Source: CAD feature listing. Evaluate the final solid. Frame: model axes, mm. A direction names the side the tool comes from. Give positions to 0.01 mm unless a question says otherwise; leave off trailing zeros. Order: outer loops, then holes, each group sorted by start corner. A loop starts at its lowest first (then second) coordinate and runs counter-clockwise, first axis right, second up. Notation, with made-up numbers: M -38,71 L 3,71 A19 cw 3,103 Z; hole C 79,81.25 d3. An arc over 180 degrees is marked long. One line per question, with ' | ' between items. Start each with the question number.
from build123d import *

# Parameters (mm, degrees)
RESSALTO_EXTRUS_O1_DEPTH = 5
ESBO_O2_R                = 1.5
CORTE_EXTRUS_O1_DEPTH    = 5
FILETE1_R                = 10
CORTE_EXTRUS_O2_DEPTH    = 5
FILETE2_R                = 5


with BuildPart() as part:
    # Esboço1 → Ressalto-extrusão1 (new body)
    with BuildSketch(Plane.XY):
        with BuildLine():
            Line((-14.089663978, 13.135393664), (-14.089663978, 28.135393664))
            Line((-14.089663978, 28.135393664), (-34.089663978, 28.135393664))
            Line((-34.089663978, 28.135393664), (-34.089663978, 128.135393664))
            Line((-34.089663978, 128.135393664), (25.910336022, 128.135393664))
            Line((25.910336022, 128.135393664), (25.910336022, 28.135393664))
            Line((25.910336022, 28.135393664), (5.910336022, 28.135393664))
            Line((5.910336022, 28.135393664), (5.910336022, 13.135393664))
            ThreePointArc((5.910336022, 13.135393664), (-4.089663978, 3.135393664), (-14.089663978, 13.135393664))
        make_face()
    extrude(amount=RESSALTO_EXTRUS_O1_DEPTH)

    # Esboço2 → Corte-extrusão1 (cut)
    with BuildSketch(Plane.XY.offset(5)):
        with Locations((-4.089663978, 13.135393664)):
            Circle(ESBO_O2_R)
    extrude(amount=-CORTE_EXTRUS_O1_DEPTH, mode=Mode.SUBTRACT)

    # Filete1
    filete1_edges = [part.edges().sort_by_distance(p)[0] for p in [
        (5.910336022, 28.135393664, 2.5),
        (-14.089663978, 28.135393664, 2.5),
    ]]
    fillet(filete1_edges, radius=FILETE1_R)
    filete1_2_edges = [part.edges().sort_by_distance(p)[0] for p in [
        (25.910336022, 28.135393664, 2.5),
        (-34.089663978, 28.135393664, 2.5),
    ]]
    fillet(filete1_2_edges, radius=FILETE1_R - 0.0001)  # a hair under: the kernel refuses the full size

    # Esboço3 → Corte-extrusão2 (cut)
    with BuildSketch(Plane.XY.offset(5)):
        with BuildLine():
            ThreePointArc((-34.089663978, 38.135393664), (-27.631189305, 83.135393664), (-34.089663978, 128.135393664))
            Line((-34.089663978, 128.135393664), (-34.089663978, 38.135393664))
        make_face()
        with BuildLine():
            ThreePointArc((25.910336022, 38.135393664), (19.45186135, 83.135393664), (25.910336022, 128.135393664))
            Line((25.910336022, 128.135393664), (25.910336022, 38.135393664))
        make_face()
    extrude(amount=-CORTE_EXTRUS_O2_DEPTH, mode=Mode.SUBTRACT)

    # Filete2
    filete2_edges = [part.edges().sort_by_distance(p)[0] for p in [
        (-34.089663978, 128.135393664, 2.5),
        (25.910336022, 128.135393664, 2.5),
    ]]
    fillet(filete2_edges, radius=FILETE2_R)


solid = part.part
Item 1: Pin query (flat end, axial travel): pin 1 Ø3.5 at (x, y) = (-4.09, 13.14) entering from -Z; pin 2 Ø3 at (y, z) = (55, 1.5) entering from -X. Return the tip coordinate at first contact, or that it passes through.
Item 2: Cut plane D-D on x = 9.5. Return the cut outline in (y, z).
Item 3: Mould query, pull axis Y, two halves, no side actions, for faces 4 (the flat face through (-4, 80, 0)), 5 (the cylindrical face through (-27.677, 79.324, 2.535)), 6 (the cylindrical face through (-31.083, 30.987, 2.535)), 7 (the cylindrical face through (19.497, 79.324, 2.535)). Classes: pulls with the +Y half, pulls with the -Y half, needs draft (parallel to the pull), parting line crosses it, or undercut.
Item 4: Reachability of faces 1 (the flat face through (5.91, 16, 2)), 2 (the flat face through (-4, 128.135, 2)), 3 (the flat face through (-14.09, 16, 2)) from +Z, -Z, +X, -X, +Y, -Y: full face, straight path, thin tool, end or side. Return the list, or none.
Item 5: Cut plane C-C on y = 108. Return the cut outline in (x, z), and give its area (3 significant figures).
Item 6: Line query: line 1 (X direction, y = 18, z = 4.75); line 2 (Y direction, x = -3.5, z = 1.95); line 3 (Y direction, x = 10, z = 3.4). Output: solid intervals per line, ascending.
Item 7: Cut plane A-A on x = -4. Return the cut outline in (y, z).
Results are:
1) pin 1: stops at z = 0 | pin 2: stops at x = -30.4
2) outline: M 25.81,0 L 128.14,0 L 128.14,5 L 25.81,5 Z
3) face 4: needs draft | face 5: undercut | face 6: pulls with the -Y half | face 7: undercut
4) face 1: +Z, -Z, +X, -Y | face 2: +Z, -Z, +X, -X, +Y | face 3: +Z, -Z, -X, -Y
5) outline: M -29.58,0 L 21.4,0 L 21.4,5 L -29.58,5 Z | area: 255 mm2
6) line 1: x = -14.09 to 5.91 | line 2: y = 3.15 to 11.76, 14.51 to 128.14 | line 3: y = 26.2 to 128.14
7) outline: M 3.14,0 L 11.64,0 L 11.64,5 L 3.14,5 Z; M 14.63,0 L 128.14,0 L 128.14,5 L 14.63,5 Z
